Here's the drawing with two shaded views (mm, measured from the low corner). I have some questions. A direction names the side the tool comes from. Give positions to 0.01 mm unless a question says otherwise; leave off trailing zeros. Loops run counter-clockwise (first coordinate to the right, second up) from the corner with the lowest first, then second, coordinate; pieces in that order, holes last. Notation, with made-up numbers: M 53,33 L 99,33 A25 cw 99,53 Z; hole C 32,-25.5 d1. An arc over 180 degrees is marked long. Write item = value, one per line. Start each with the question number.
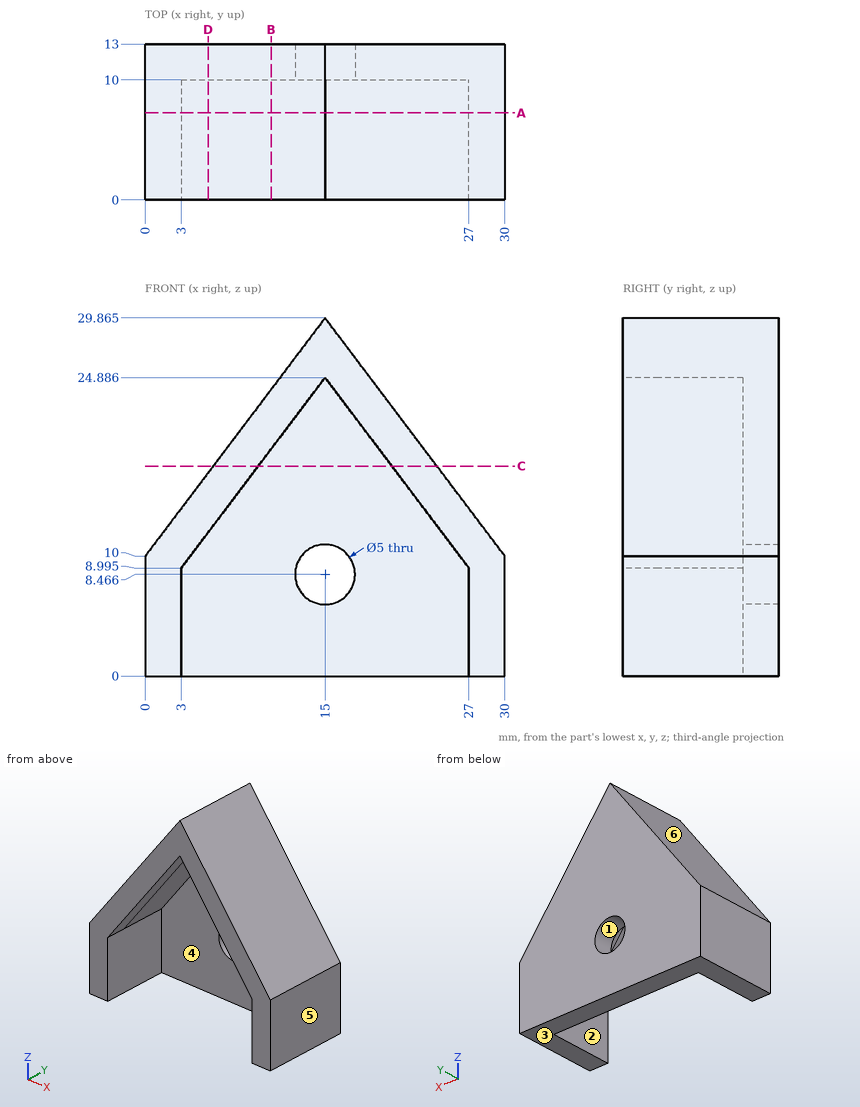
Q1. We'd pull the mould along X, two halves only. Please class the marked faces 3, 4, 5 and 6: pulls with the +X half, pulls with the -X half, needs draft (parallel to the pull), parting line crosses it, or undercut.
Q2. If we section it at A-A, the plane y = 7.25: List the corners of the cut face in (x, z) for me (1 decimal).
Q3. If I drill on line 1 along X through (y, z) = (2, 9) (1 decimal); line 2 along Y through (x, z) = (8.5, 5); line 3 along X through (y, z) = (1.25, 16.25), over which ranges is the centre line in solid material (lowest first)?
Q4. Will these pins go through, and if not, where does the flat tip stop? pin 1 (6 mm diameter, centred on x = 18, z = 10, fed in from -Y); pin 2 (4 mm diameter, centred on y = 9, z = 13.5, fed in from -X); pin 3 (1.5 mm diameter, centred on y = 4, z = 16, fed in from -X) (1 decimal); pin 4 (4.5 mm diameter, centred on x = 15, z = 8.47, fed in from -Y).
Q5. If we section it at B-B, the plane x = 10.5: List the corners of the cut face in (y, z) for me (1 decimal).
Q6. On a 3-axis mill with a long thin cutter (end or side, diameter ignored), from which of +Z, -Z, +X, -X, +Y, -Y can I reach the whole of each face in a straight line? I mean the marked faces 1 and 2. Say none if no direction works.
Q7. If we section it at C-C, the plane z = 17.5: List the corners of the cut face in (x, y) for me, then the cut area to 3 significant figures.
Q8. If we section it at D-D, the plane x = 5.25: List the corners of the cut face in (y, z) for me (1 decimal), then the cut area to 3 significant figures.
Resolved:
q1.face_3 = needs draft
q1.face_4 = undercut
q1.face_5 = pulls with the +X half
q1.face_6 = pulls with the -X half
q2.outline = M 0,0 L 3,0 L 3,9 L 15,24.9 L 27,9 L 27,0 L 30,0 L 30,10 L 15,29.9 L 0,10 Z
q3.line_1 = 0 to 3, 27 to 30
q3.line_2 = 10 to 13
q3.line_3 = 4.72 to 8.48, 21.52 to 25.28
q4.pin_1 = 10
q4.pin_2 = 1.13
q4.pin_3 = 4
q4.pin_4 = through
q5.outline = M 0,18.9 L 10,18.9 L 10,0 L 13,0 L 13,23.9 L 0,23.9 Z
q6.face_1 = +Y, -Y
q6.face_2 = -Z, -Y
q7.outline = M 5.66,0 L 9.42,0 L 9.42,10 L 20.58,10 L 20.58,0 L 24.34,0 L 24.34,13 L 5.66,13 Z
q7.area = 131 mm²
q8.outline = M 0,12 L 10,12 L 10,0 L 13,0 L 13,17 L 0,17 Z
q8.area = 101 mm²
